Can you work these out from the model? Positions are in its coordinate system, mm. A direction names the side the tool comes from. Round coordinates to 2 decimals unless told otherwise and drop trailing zeros. Loops run counter-clockwise (first coordinate to the right, second up) from the corner with the lowest first, then second, coordinate; pieces in that order, holes last. Notation, with made-up numbers: (-1, -10) -> (13, -10) arc R21 ccw to (13, 13) -> close; hole circle Ø8 at (34, -1). An arc over 180 degrees is marked (long way). Answer as a JSON object with one key per item and string values.
```python
from build123d import *

# Parameters (mm, degrees)
BOSS_EXTRU_1_DEPTH = 5
ESQUISSE2_R        = 1.5
ESQUISSE2_R_2      = 1
BOSS_EXTRU_2_DEPTH = 5
CONG_1_R           = 10


with BuildPart() as part:
    # Esquisse1 → Boss.-Extru.1 (new body)
    with BuildSketch(Plane.XY):
        Polygon((-12.911051911, 37.825067336), (-12.911051911, -4.674932664), (-6.211051911, -4.674932664), (-6.211051911, 0.325067336), (-4.511051911, 0.325067336), (-4.511051911, 2.321763371), (-5.761051911, 2.321763371), (-5.761051911, 5.321763371), (-4.511051911, 5.321763371), (-4.511051911, 9.575067336), (-1.311051911, 9.575067336), (-1.311051911, 5.321763371), (-0.061051911, 5.321763371), (-0.061051911, 2.321763371), (-1.311051911, 2.321763371), (-1.311051911, 0.325067336), (0.388948089, 0.325067336), (0.388948089, -4.674932664), (7.088948089, -4.674932664), (7.088948089, 37.825067336), (0.388948089, 37.825067336), (0.388948089, 32.825067336), (-1.311051911, 32.825067336), (-1.311051911, 30.828371301), (-0.061051911, 30.828371301), (-0.061051911, 27.828371301), (-1.311051911, 27.828371301), (-1.311051911, 23.575067336), (-4.511051911, 23.575067336), (-4.511051911, 27.828371301), (-5.761051911, 27.828371301), (-5.761051911, 30.828371301), (-4.511051911, 30.828371301), (-4.511051911, 32.825067336), (-6.211051911, 32.825067336), (-6.211051911, 37.825067336), align=None)
    extrude(amount=BOSS_EXTRU_1_DEPTH)

    # Esquisse2 → Boss.-Extru.2 (add)
    with BuildSketch(Plane(origin=(0, 0, 0), x_dir=(-1, 0, 0), z_dir=(0, 0, -1))):
        with BuildLine():
            Line((30.411051911, 26.575067336), (12.911051911, 26.575067336))
            Line((12.911051911, 26.575067336), (12.911051911, 6.575067336))
            Line((12.911051911, 6.575067336), (30.411051911, 6.575067336))
            ThreePointArc((30.411051911, 6.575067336), (40.411051911, 16.575067336), (30.411051911, 26.575067336))
        make_face()
        with Locations((30.411051911, 16.575067336)):
            Circle(ESQUISSE2_R, mode=Mode.SUBTRACT)
        with Locations((30.411051911, 23.575067336)):
            Circle(ESQUISSE2_R_2, mode=Mode.SUBTRACT)
        with Locations((23.411051911, 16.575067336)):
            Circle(ESQUISSE2_R_2, mode=Mode.SUBTRACT)
        with Locations((30.411051911, 9.575067336)):
            Circle(ESQUISSE2_R_2, mode=Mode.SUBTRACT)
        with Locations((37.411051911, 16.575067336)):
            Circle(ESQUISSE2_R_2, mode=Mode.SUBTRACT)
    extrude(amount=-BOSS_EXTRU_2_DEPTH)

    # Congé1
    cong_1_edges = [part.edges().sort_by_distance(p)[0] for p in [
        (-12.911051911, 26.575067336, 2.5),
        (-12.911051911, 6.575067336, 2.5),
    ]]
    fillet(cong_1_edges, radius=CONG_1_R)


solid = part.part
```
Q1. I want a section at B-B, the plane x = -37. Write out the boundary of the cut face in (y, z), then the cut area to 3 significant figures.
Determined:
{"outline": "(9.05, 0) -> (15.66, 0) -> (15.66, 5) -> (9.05, 5) -> close; (17.49, 0) -> (24.1, 0) -> (24.1, 5) -> (17.49, 5) -> close", "area": "66.1 mm²"}
Q2. I want a section at C-C, the plane x = -25. Write out the boundary of the cut face in (y, z).
Determined:
{"outline": "(6.58, 0) -> (26.58, 0) -> (26.58, 5) -> (6.58, 5) -> close"}
Q3. We'd pull the mould along X, two halves only. Please class faces 1 (the cylindrical face through (-15.763, 3.568, 2.535)), 2 (the flat face through (4, -4.675, 2)), 3 (the flat face through (-3, 23.575, 2)): pulls with the +X half, pulls with the -X half, needs draft (parallel to the pull), parting line crosses it, or undercut.
Determined:
{"face 1": "pulls with the -X half", "face 2": "needs draft", "face 3": "undercut"}
Q4. On a 3-axis mill with a long thin cutter (end or side, diameter ignored), from which of +Z, -Z, +X, -X, +Y, -Y can I reach the whole of each face in a straight line? I mean faces 4 (the flat face through (-12.911, -4, 2)), 5 (the flat face through (-4.511, 1, 2)), 6 (the cylindrical face through (-15.763, 29.582, 2.535)), 7 (the flat face through (-5, 30.828, 2)), 8 (the flat face through (-5, 32.825, 2)). Say none if no direction works.
Determined:
{"face 4": "+Z, -Z, -X, -Y", "face 5": "+Z, -Z, -Y", "face 6": "+Z, -Z, -X, +Y", "face 7": "+Z, -Z", "face 8": "+Z, -Z, +Y"}
Q5. I want a section at A-A, the plane y = 1.5. Write out the boundary of the cut face in (x, z).
Determined:
{"outline": "(-14.21, 0) -> (-4.51, 0) -> (-4.51, 5) -> (-14.21, 5) -> close; (-1.31, 0) -> (7.09, 0) -> (7.09, 5) -> (-1.31, 5) -> close"}
Q6. I want a section at D-D, the plane z = 3.9. Give the number of separate pieces and of enclosed holes in the cut face, then the cut area to 3 significant figures.
Determined:
{"separate pieces": "1", "enclosed holes": "5", "area": "1,240 mm²"}
Q7. If I drill on L1, parallel to Y at x = -1, z = 0.9; L2, parallel to X at y = 16.5, z = 3.5; L3, parallel to Y at x = -2, z = 1.1, over which ranges is the centre line in solid material (lowest first)? Write a range as [from, to].
Determined:
{"L1": "[0.33, 2.32], [5.32, 27.83], [30.83, 32.83]", "L2": "[-40.41, -38.41], [-36.41, -31.91], [-28.91, -24.41], [-22.41, 7.09]", "L3": "[9.58, 23.58]"}
Q8. I'm going to push flat-ended pins straight in: pin 1 (0.6 mm diameter, centred on x = -0.5, z = 2.5, fed in from +Y); pin 2 (1.6 mm diameter, centred on x = -3.5, z = 2.5, fed in from -Y); pin 3 (0.9 mm diameter, centred on y = 4, z = 2.5, fed in from -X). Where does each tip first touch, or does it pass through?
Determined:
{"pin 1": "y = 32.83", "pin 2": "y = 9.58", "pin 3": "x = -16.75"}
